Read the model definition and answer for the solid it produces. Units are mm, in the model's axes. A direction names the side the tool comes from. Give positions to 0.01 mm unless a question says otherwise; leave off trailing zeros. Order: outer loops, then holes, each group sorted by start corner. A loop starts at its lowest first (then second) coordinate and runs counter-clockwise, first axis right, second up.
```python
from build123d import *

# Parameters (mm, degrees)
SKETCH1_W                    = 290
SKETCH1_H                    = 0.7366
BASE_FLANGE1_DEPTH           = 35
EDGE_FLANGE1_STRIP_W         = 12.9464
EDGE_FLANGE1_STRIP_H         = 0.7366
EDGE_FLANGE1_STRIP_CUT_DEPTH = 290
EDGE_FLANGE1_DEPTH           = 290
SKETCH11_R                   = 5
CUT_EXTRUDE1_DEPTH           = 153.931874309
LPATTERN1_COUNT              = 14
LPATTERN1_PITCH              = 80
SKETCH12_R                   = 5
CUT_EXTRUDE2_DEPTH           = 35
LPATTERN2_COUNT              = 15
LPATTERN2_PITCH              = 80


# Sheet-metal steps are written as plain solids
with BuildPart() as part:
    # Sketch1 → Base-Flange1 (new body)
    with BuildSketch(Plane(origin=(0, 0, 0), x_dir=(1, 0, 0), z_dir=(0, 1, 0))):
        with Locations((0, -0.3683)):
            Rectangle(SKETCH1_W, SKETCH1_H)
    extrude(amount=BASE_FLANGE1_DEPTH)

    # Edge-Flange1 strip (across the edge) → Edge-Flange1 strip cut (cut)
    with BuildSketch(Plane(origin=(145, 35, 0.7366), x_dir=(0, -1, 0), z_dir=(-1, 0, 0))):
        with Locations((-0.7366, -0.3683)):
            Rectangle(EDGE_FLANGE1_STRIP_W, EDGE_FLANGE1_STRIP_H)
    extrude(amount=EDGE_FLANGE1_STRIP_CUT_DEPTH, mode=Mode.SUBTRACT)

    # Edge-Flange1 section (across the edge) → Edge-Flange1 (add)
    with BuildSketch(Plane(origin=(145, 35, 0.7366), x_dir=(0, -1, 0), z_dir=(-1, 0, 0))):
        with BuildLine():
            Line((0, 5), (0, 33))
            Line((0, 33), (0.7366, 33))
            Line((0.7366, 33), (0.7366, 5))
            ThreePointArc((0.7366, 5), (2.201066094, 1.464466094), (5.7366, 0))
            Line((5.7366, 0), (5.7366, -0.7366))
            ThreePointArc((5.7366, -0.7366), (1.680211239, 0.943611239), (0, 5))
        make_face()
    extrude(amount=EDGE_FLANGE1_DEPTH)

    # Sketch11 → Cut-Extrude1 (cut, through all)
    with BuildSketch(Plane(origin=(0, 35, 0), x_dir=(1, 0, 0), z_dir=(0, 1, 0))):
        with Locations((145, -20.7366)):
            Circle(SKETCH11_R)
        with BuildLine():
            Line((129, -25.7366), (121, -25.7366))
            ThreePointArc((121, -25.7366), (116, -20.7366), (121, -15.7366))
            Line((121, -15.7366), (129, -15.7366))
            ThreePointArc((129, -15.7366), (134, -20.7366), (129, -25.7366))
        make_face()
        with BuildLine():
            Line((89, -25.7366), (81, -25.7366))
            ThreePointArc((81, -25.7366), (76, -20.7366), (81, -15.7366))
            Line((81, -15.7366), (89, -15.7366))
            ThreePointArc((89, -15.7366), (94, -20.7366), (89, -25.7366))
        make_face()
        with BuildLine():
            Line((100, -23.4866), (100, -17.9866))
            ThreePointArc((100, -17.9866), (105, -12.9866), (110, -17.9866))
            Line((110, -17.9866), (110, -23.4866))
            ThreePointArc((110, -23.4866), (105, -28.4866), (100, -23.4866))
        make_face()
    cut_extrude1 = extrude(amount=-CUT_EXTRUDE1_DEPTH, mode=Mode.SUBTRACT)

    # LPattern1: Cut-Extrude1 ×14
    with Locations(*[(-i * LPATTERN1_PITCH, 0, 0) for i in range(1, LPATTERN1_COUNT)]):
        add(cut_extrude1, mode=Mode.SUBTRACT)

    # Sketch12 → Cut-Extrude2 (cut)
    with BuildSketch(Plane.XY.offset(0.7366)):
        with Locations((145, 13)):
            Circle(SKETCH12_R)
        with BuildLine():
            Line((129, 8), (121, 8))
            ThreePointArc((121, 8), (116, 13), (121, 18))
            Line((121, 18), (129, 18))
            ThreePointArc((129, 18), (134, 13), (129, 8))
        make_face()
        with BuildLine():
            Line((100, 10.25), (100, 15.75))
            ThreePointArc((100, 15.75), (105, 20.75), (110, 15.75))
            Line((110, 15.75), (110, 10.25))
            ThreePointArc((110, 10.25), (105, 5.25), (100, 10.25))
        make_face()
        with BuildLine():
            Line((89, 8), (81, 8))
            ThreePointArc((81, 8), (76, 13), (81, 18))
            Line((81, 18), (89, 18))
            ThreePointArc((89, 18), (94, 13), (89, 8))
        make_face()
    cut_extrude2 = extrude(amount=-CUT_EXTRUDE2_DEPTH, mode=Mode.SUBTRACT)

    # LPattern2: Cut-Extrude2 ×15
    with Locations(*[(-i * LPATTERN2_PITCH, 0, 0) for i in range(1, LPATTERN2_COUNT)]):
        add(cut_extrude2, mode=Mode.SUBTRACT)


solid = part.part
```
1) Given pin 1 (0.8 mm diameter, centred on x = 83.5, y = 34.5, fed in from -Z); pin 2 (9 mm diameter, centred on x = -95, y = 13, fed in from +Z); pin 3 (2 mm diameter, centred on x = 29.5, z = 4.5, fed in from +Y); pin 4 (0.6 mm diameter, centred on y = 34.5, z = 20, fed in from +X), each flat-ended and moving along its own axis, determine where each tip first touches the part or whether it passes through.
Final values:
pin 1: stops at z = 2.65
pin 2: passes through
pin 3: stops at y = 35
pin 4: stops at x = 140.11
2) The part is cut by section B-B on x = -103. Determine the outline of the cut face in (y, z), and give its area (3 significant figures).
Final values:
outline: (0, 0) - (29.26, 0) arc R5.74 ccw to (35, 5.74) - (35, 33.74) - (34.26, 33.74) - (34.26, 5.74) arc R5 cw to (29.26, 0.74) - (0, 0.74) - close
area: 48.4 mm2
3) Consider L1, parallel to Z at x = -118, y = 1; L2, parallel to Y at x = 21, z = 31.5; L3, parallel to Z at x = -56, y = 30. Determine where each line is inside the solid, lowest interval first.
Final values:
L1: z = 0 to 0.74
L2: y = 34.26 to 35
L3: z = 0.05 to 0.79
4) A tool of negligible diameter and unlimited length cuts with its end or side. For faces 5 (the face through (-2, 18, 0.737)), 6 (the face through (-4, 34.6, 20.8)), 7 (the face through (-135.11, 20.75, 0.37)), from which of +Z, -Z, +X, -X, +Y, -Y can it reach the whole face along a straight path? Write none if from no direction.
Final values:
face 5: +Z, +X, -X, -Y
face 6: +Y, -Y
face 7: +Z, -Z
5) For a pull along X with two mould halves and no side action, classify faces 1 (the face through (145, 33, 2)), 2 (the face through (2, 34.263, 14)), 3 (the face through (134, 34.6, 20.6)), 4 (the face through (14, 34.6, 20.6)) as released by +X, released by -X, zero draft, split by the parting line, or undercut.
Final values:
face 1: released by +X
face 2: zero draft
face 3: undercut
face 4: undercut
6) The part is cut by section C-C on y = 13. Count the separate pieces of the cut face and the enclosed holes in it, and give its area (3 significant figures).
Final values:
separate pieces: 15
enclosed holes: 0
area: 65.6 mm2
7) The part is cut by section A-A on x = 25. Determine the outline of the cut face in (y, z), and give its area (3 significant figures).
Final values:
outline: (0, 0) - (5.25, 0) - (5.25, 0.74) - (0, 0.74) - close; (20.75, 0) - (29.26, 0) arc R5.74 ccw to (35, 5.74) - (35, 12.99) - (34.26, 12.99) - (34.26, 5.74) arc R5 cw to (29.26, 0.74) - (20.75, 0.74) - close; (34.26, 28.49) - (35, 28.49) - (35, 33.74) - (34.26, 33.74) - close
area: 25.6 mm2
8) The part is cut by section D-D on x = 85. Determine the outline of the cut face in (y, z), and give its area (3 significant figures).
Final values:
outline: (0, 0) - (8, 0) - (8, 0.74) - (0, 0.74) - close; (18, 0) - (29.26, 0) arc R5.74 ccw to (35, 5.74) - (35, 15.74) - (34.26, 15.74) - (34.26, 5.74) arc R5 cw to (29.26, 0.74) - (18, 0.74) - close; (34.26, 25.74) - (35, 25.74) - (35, 33.74) - (34.26, 33.74) - close
area: 33.7 mm2
